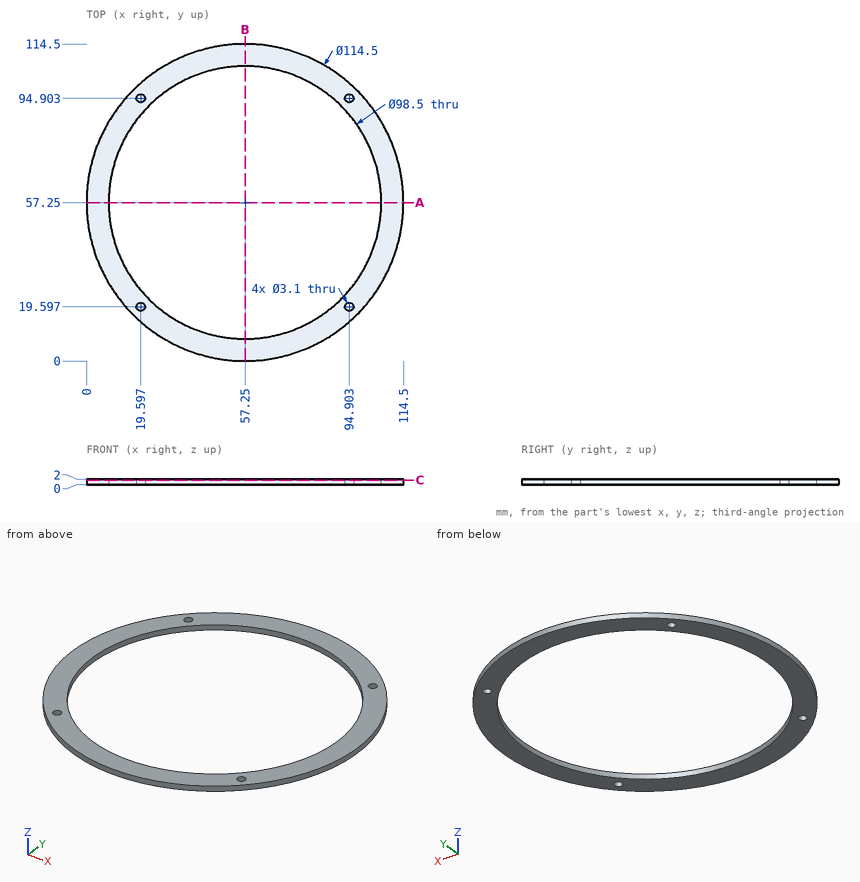
The drawing under review shows one solid part. Ordinate dimensions are in mm from its lowest x, y, z. Coordinates: 2 decimals unless noted, no trailing zeros. Write each loop counter-clockwise with the first axis right and the second up, starting at its lowest first coordinate (ties: lowest second). Pieces come first, ordered by that corner, then holes. Notation, with made-up numbers: (28, -2) - (39, -2) arc R22 cw to (39, 34) - close; hole circle Ø9 at (72, 83). An arc over 180 degrees is marked (long way). Answer as CSV lines item,"result".
(1) We need section C-C (z = 1.6). Give the boundary of the cut face in (x, y), plus the area to 3 significant figures.
Data:
outline,"circle Ø114.5 at (57.25, 57.25); hole circle Ø98.5 at (57.25, 57.25); hole circle Ø3.1 at (19.6, 19.6); hole circle Ø3.1 at (19.6, 94.9); hole circle Ø3.1 at (94.9, 19.6); hole circle Ø3.1 at (94.9, 94.9)"
area,"2,650 mm2"
(2) We need section A-A (y = 57.25). Give the boundary of the cut face in (x, z), plus the area to 3 significant figures.
Data:
outline,"(0, 0) - (8, 0) - (8, 2) - (0, 2) - close; (106.5, 0) - (114.5, 0) - (114.5, 2) - (106.5, 2) - close"
area,"32.0 mm2"
(3) For line 1 along Y through (x, z) = (58, 0.4) (1 decimal); line 2 along X through (y, z) = (43, 0.3); line 3 along Y through (x, z) = (29, 1.4) (1 decimal), list the stretches that pass through material, from the lowest coordinate up. Write a range as [from, to].
Data:
line 1,"y = [0, 8], [106.5, 114.5]"
line 2,"x = [1.8, 10.11], [104.39, 112.7]"
line 3,"y = [7.5, 16.9], [97.6, 107]"
(4) Clearance check with flat-ended pins moving along their axes: pin 1 Ø10 at (x, y) = (26.5, 22.5) entering from +Z; pin 2 Ø1 at (y, z) = (45.5, 1.5) entering from +X; pin 3 Ø1 at (y, z) = (19, 0.5) entering from -X. State where each tip first meets the part, or that it passes through.
Data:
pin 1,"stops at z = 2"
pin 2,"stops at x = 113.38"
pin 3,"stops at x = 14.21"
